```python
from build123d import *

# Parameters (mm, degrees)
BOSS_EXTRU_1_DEPTH      = 6
ESQUISSE2_R             = 4.5
ENL_V_MAT_EXTRU_1_DEPTH = 708.132236572
ESQUISSE5_R             = 2.5
ENL_V_MAT_EXTRU_3_DEPTH = 708.132236572
CHANFREIN2_SIZE         = 2


with BuildPart() as part:
    # Esquisse1 → Boss.-Extru.1 (new body)
    with BuildSketch(Plane.XY):
        Polygon((0, 0), (0, 48), (452, 500), (500, 500), (500, 0), align=None)
    extrude(amount=BOSS_EXTRU_1_DEPTH)

    # Esquisse2 → Enlèv. mat.-Extru.1 (cut, through all)
    with BuildSketch(Plane.XY.offset(6)):
        with Locations((24, 18)):
            Circle(ESQUISSE2_R)
        with Locations((250, 18)):
            Circle(ESQUISSE2_R)
        with Locations((476, 18)):
            Circle(ESQUISSE2_R)
        with Locations((482, 483)):
            Circle(ESQUISSE2_R)
        with Locations((482, 317)):
            Circle(ESQUISSE2_R)
    extrude(amount=-ENL_V_MAT_EXTRU_1_DEPTH, mode=Mode.SUBTRACT)

    # Esquisse5 → Enlèv. mat.-Extru.3 (cut, through all)
    with BuildSketch(Plane.XY.offset(6)):
        with Locations((165.188816818, 179.247691321)):
            Circle(ESQUISSE5_R)
        with Locations((320.752308679, 334.811183182)):
            Circle(ESQUISSE5_R)
        with Locations((102.970562748, 24)):
            Circle(ESQUISSE5_R)
        with Locations((382.970562748, 24)):
            Circle(ESQUISSE5_R)
        with Locations((476, 397.029437252)):
            Circle(ESQUISSE5_R)
        with Locations((476, 117.029437252)):
            Circle(ESQUISSE5_R)
    extrude(amount=-ENL_V_MAT_EXTRU_3_DEPTH, mode=Mode.SUBTRACT)

    # Chanfrein2
    chanfrein2_edges = [part.edges().sort_by_distance(p)[0] for p in [
        (318.252308679, 334.811183182, 0),
        (100.470562748, 24, 0),
        (380.470562748, 24, 0),
        (473.5, 397.029437252, 0),
        (473.5, 117.029437252, 0),
        (162.688816818, 179.247691321, 0),
    ]]
    chamfer(chanfrein2_edges, length=CHANFREIN2_SIZE)


solid = part.part
```
Can you work these out from the model? Positions are in its coordinate system, mm. Give positions to 0.01 mm unless a question says otherwise; leave off trailing zeros. Order: outer loops, then holes, each group sorted by start corner. A loop starts at its lowest first (then second) coordinate and runs counter-clockwise, first axis right, second up. Notation, with made-up numbers: (-16.5, 62.5) - (33.5, 62.5) arc R17 cw to (33.5, 83.5) - close; hole circle Ø8 at (26.5, -10.5). An arc over 180 degrees is marked (long way). Use a Markdown table: item, result. Add a question column.
Q1. If we section it at C-C on x = 359.5: Write out the boundary of the cut face in (y, z).
Q2. If we section it at B-B on z = 4.9: Count the separate pieces of the cut face and the enclosed holes in it, plus the area to 3 significant figures.
Q3. If we section it at A-A on y = 371: Write out the boundary of the cut face in (x, z).
Q4. Please list where these lines run through material, in increasing order: line 1 along Y through (x, z) = (476, 3.15); line 2 along Y through (x, z) = (482, 2.1); line 3 along X through (y, z) = (179.5, 3.2).
Q5. I'm going to push flat-ended pins straight in: pin 1 (4.5 mm diameter, centred on x = 476, y = 397.03, fed in from -Z); pin 2 (6 mm diameter, centred on x = 165.19, y = 179.25, fed in from -Z); pin 3 (2 mm diameter, centred on x = 196, z = 5.5, fed in from +Y). Where does each tip first touch, or does it pass through?
Answers follow:
| question | item | result |
|---|---|---|
| 1 | outline | (0, 0) - (407.5, 0) - (407.5, 6) - (0, 6) - close |
| 2 | separate pieces | 1 |
| 2 | enclosed holes | 11 |
| 2 | area | 147,000 mm^2 |
| 3 | outline | (323, 0) - (500, 0) - (500, 6) - (323, 6) - close |
| 4 | line 1 | y = 0 to 13.5, 22.5 to 114.53, 119.53 to 394.53, 399.53 to 500 |
| 4 | line 2 | y = 0 to 312.5, 321.5 to 478.5, 487.5 to 500 |
| 4 | line 3 | x = 131.5 to 162.7, 167.68 to 500 |
| 5 | pin 1 | passes through |
| 5 | pin 2 | stops at z = 1.5 |
| 5 | pin 3 | stops at y = 245 |
